Can you work these out from the drawing? Everything is in mm from the part's minimum corner. Give positions to 0.01 mm unless a question says otherwise; leave off trailing zeros. Loops run counter-clockwise (first coordinate to the right, second up) from the corner with the lowest first, then second, coordinate; pieces in that order, holes last. Notation, with made-up numbers: (6, 11.5) - (33, 11.5) arc R18 cw to (33, 37.5) - close; hole circle Ø11 at (13.5, 4). An arc over 180 degrees is marked (long way). Answer in a Markdown table with one row per item.
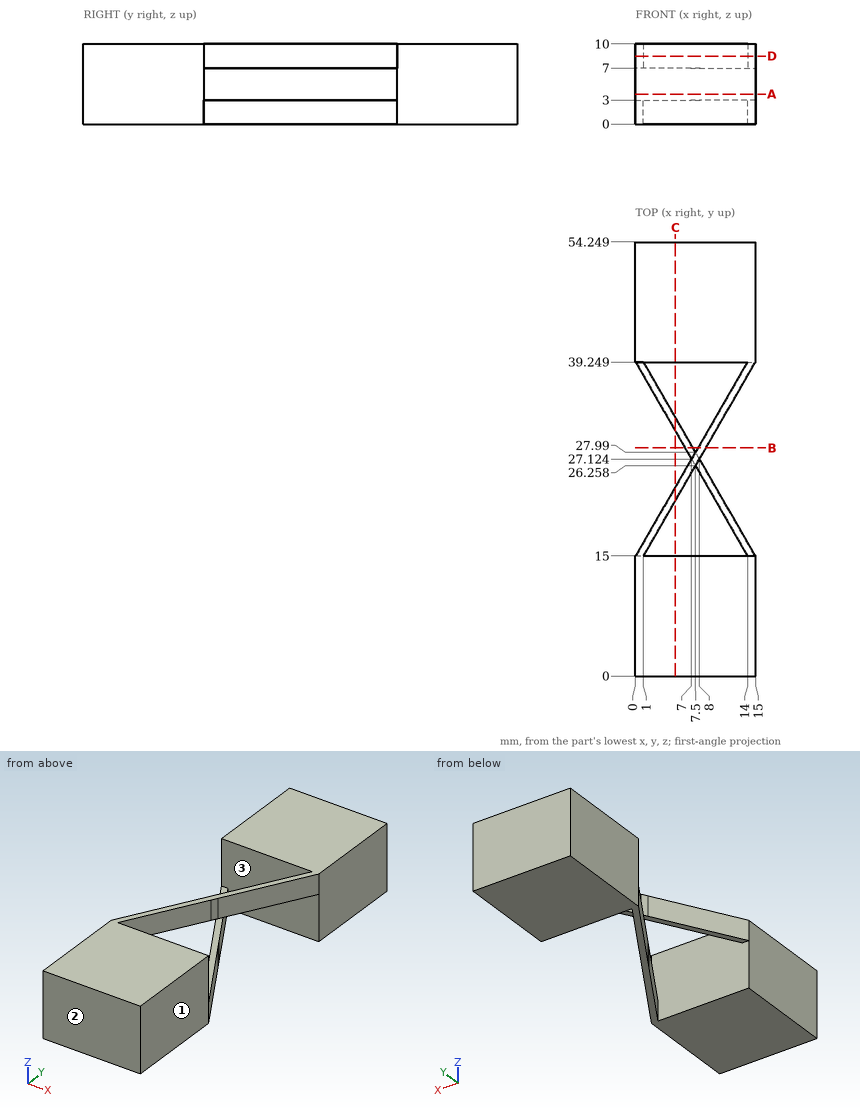
Q1. Imagine slicing it at D-D, the plane z = 8.5. Write out the boundary of the cut face in (x, y) (1 decimal), and give its area (3 significant figures).
Checked values:
| item | result |
|---|---|
| outline | (0, 0) - (15, 0) - (15, 15) - (1, 15) - (15, 39.2) - (15, 54.2) - (0, 54.2) - (0, 39.2) - (14, 39.2) - (0, 15) - close |
| area | 474 mm² |
Q2. Imagine slicing it at C-C, the plane x = 5. Write out the boundary of the cut face in (y, z), and give its area (3 significant figures).
Checked values:
| item | result |
|---|---|
| outline | (0, 0) - (15, 0) - (15, 10) - (0, 10) - close; (21.93, 7) - (23.66, 7) - (23.66, 10) - (21.93, 10) - close; (30.59, 0) - (32.32, 0) - (32.32, 3) - (30.59, 3) - close; (39.25, 0) - (54.25, 0) - (54.25, 10) - (39.25, 10) - close |
| area | 310 mm² |
Q3. For pin 1 (1 mm diameter, centred on y = 24, z = 2.5, fed in from -X) (1 decimal); pin 2 (1.5 mm diameter, centred on y = 23, z = 4.5, fed in from +X), each with a flat end and sliding along its axis, tell me the tip position at first contact or that it passes through.
Checked values:
| item | result |
|---|---|
| pin 1 | stops at x = 8.5 |
| pin 2 | passes through |
Q4. If I drill on line 1 (Y direction, x = 2.25, z = 5.5); line 2 (Y direction, x = 8.25, z = 1.5); line 3 (Z direction, x = 6.75, y = 29), over which ranges is the centre line in solid material (lowest first)? Write a range as [from, to].
Checked values:
| item | result |
|---|---|
| line 1 | y = [0, 15], [39.25, 54.25] |
| line 2 | y = [0, 15], [24.96, 26.69], [39.25, 54.25] |
| line 3 | z = [0, 3] |
Q5. Imagine slicing it at A-A, the plane z = 3.75. Write out the boundary of the cut face in (x, y).
Checked values:
| item | result |
|---|---|
| outline | (0, 0) - (15, 0) - (15, 15) - (0, 15) - close; (0, 39.25) - (15, 39.25) - (15, 54.25) - (0, 54.25) - close |
Q6. Imagine slicing it at B-B, the plane y = 28.5. Write out the boundary of the cut face in (x, z) (1 decimal).
Checked values:
| item | result |
|---|---|
| outline | (6.2, 0) - (7.2, 0) - (7.2, 3) - (6.2, 3) - close; (7.8, 7) - (8.8, 7) - (8.8, 10) - (7.8, 10) - close |
Q7. If we mould it in two halves opening along Y, with no side actions, what happens to the marked faces 1, 2 and 3? For each: released by +Y, released by -Y, zero draft, split by the parting line, or undercut.
Checked values:
| item | result |
|---|---|
| face 1 | zero draft |
| face 2 | released by -Y |
| face 3 | undercut |
